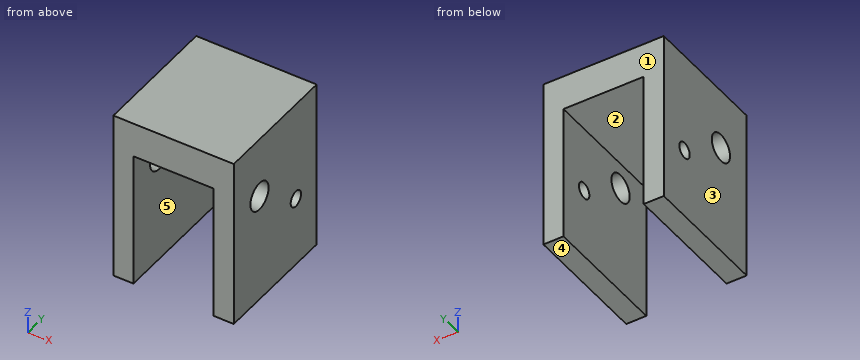
from build123d import *

# Parameters (mm, degrees)
SKETCH1_W           = 21.356696791
SKETCH1_H           = 15.93739856
SKETCH1_R           = 1.75
SKETCH1_R_2         = 1
BOSS_EXTRUDE1_DEPTH = 15
CUT_EXTRUDE1_REACH  = 17.937
SKETCH2_W           = 10
SKETCH2_H           = 17


with BuildPart() as part:
    # Sketch1 → Boss-Extrude1 (new body)
    with BuildSketch(Plane(origin=(0, 0, 0), x_dir=(0, 0, -1), z_dir=(1, 0, 0))):
        with Locations((3.081269675, 3.021892184)):
            Rectangle(SKETCH1_W, SKETCH1_H)
        Circle(SKETCH1_R, mode=Mode.SUBTRACT)
        with Locations((5, 7)):
            Circle(SKETCH1_R_2, mode=Mode.SUBTRACT)
    extrude(amount=BOSS_EXTRUDE1_DEPTH)

    # Sketch2 → Cut-Extrude1 (cut, up to next)
    with BuildSketch(Plane(origin=(0, 10.990591464, 0), x_dir=(1, 0, 0), z_dir=(0, 1, 0)), mode=Mode.PRIVATE) as cut_extrude1_sk1:
        with Locations((7.5, 5.259618071)):
            Rectangle(SKETCH2_W, SKETCH2_H)
    cut_extrude1_tool1 = extrude(cut_extrude1_sk1.sketch, amount=-CUT_EXTRUDE1_REACH, mode=Mode.PRIVATE) & part.part
    add(cut_extrude1_tool1.solids().sort_by_distance((7.5, 10.990591, -5.259618))[0], mode=Mode.SUBTRACT)


solid = part.part
Here's how the part is built. I have some questions about the finished solid (model axes, mm). Face numbers are marked on the shaded views. A direction names the side the tool comes from. Coordinates: 2 decimals unless noted, no trailing zeros. Order: outer loops, then holes, each group sorted by start corner. A loop starts at its lowest first (then second) coordinate and runs counter-clockwise, first axis right, second up. Notation, with made-up numbers: (22.5, 19.25) - (81.5, 19.25) arc R28 cw to (81.5, 46.25) - close; hole circle Ø10 at (30.5, 4). An arc over 180 degrees is marked (long way). Use CSV: the item, a comma, the result in double quotes. Start each with the question number.
1. Suppose I cut it at A-A on z = -5. List the corners of the cut face in (x, y) for me.
2. For the marked faces 4 and 5, which set-ups out of +Z, -Z, +X, -X, +Y, -Y let a thin tool reach every point of the face, with its end or its side?
3. Please list where these lines run through material, in increasing order: line 1 (X direction, y = -2.25, z = 2); line 2 (Z direction, x = 1.45, y = 0); line 3 (Y direction, x = 13, z = -5). Write a range as from..to.
4. If we mould it in two halves opening along X, with no side actions, what happens to the marked faces 1, 2 and 3? For each: +X half, -X half, draft (parallel to the pull), parting line (faces both ways), or undercut.
5. Suppose I cut it at C-C on z = -11.25. List the corners of the cut face in (x, y) for me.
6. Suppose I cut it at B-B on y = 7. List the corners of the cut face in (x, z) for me.
7. Suppose I cut it at D-D on x = 14. List the corners of the cut face in (y, z) for me.
8. I'm going to push a flat-ended pin straight in: pin 1 (1.5 mm diameter, centred on x = 9, y = -0.5, fed in from -Z). Where does the tip first touch, or does it pass through?
Output:
1,outline,"(0, -4.95) - (2.5, -4.95) - (2.5, 6) - (0, 6) - close; (0, 8) - (2.5, 8) - (2.5, 10.99) - (0, 10.99) - close; (12.5, -4.95) - (15, -4.95) - (15, 6) - (12.5, 6) - close; (12.5, 8) - (15, 8) - (15, 10.99) - (12.5, 10.99) - close"
2,face 4,"-Z, +X, -X, +Y, -Y"
2,face 5,"-Z, +Y, -Y"
3,line 1,"x = 0..2.5, 12.5..15"
3,line 2,"z = -13.76..-1.75, 1.75..7.6"
3,line 3,"y = -4.95..6, 8..10.99"
4,face 1,"draft"
4,face 2,"undercut"
4,face 3,"-X half"
5,outline,"(0, -4.95) - (2.5, -4.95) - (2.5, 10.99) - (0, 10.99) - close; (12.5, -4.95) - (15, -4.95) - (15, 10.99) - (12.5, 10.99) - close"
6,outline,"(0, -13.76) - (2.5, -13.76) - (2.5, -6) - (0, -6) - close; (0, -4) - (2.5, -4) - (2.5, 3.24) - (12.5, 3.24) - (12.5, -4) - (15, -4) - (15, 7.6) - (0, 7.6) - close; (12.5, -13.76) - (15, -13.76) - (15, -6) - (12.5, -6) - close"
7,outline,"(-4.95, -13.76) - (10.99, -13.76) - (10.99, 7.6) - (-4.95, 7.6) - close; hole circle Ø3.5 at (0, 0); hole circle Ø2 at (7, -5)"
8,pin 1,"stops at z = 3.24"
